```python
from build123d import *

# Parameters (mm, degrees)
ESQUISSE1_R                  = 1.5
BOSS_EXTRU_1_DEPTH           = 3
CONG_1_R                     = 5
ESQUISSE2_W                  = 9
ESQUISSE2_H                  = 9
BOSS_EXTRU_2_DEPTH           = 7
ESQUISSE3_R                  = 2.5
ENL_V_MAT_EXTRU_1_DEPTH      = 7
ESQUISSE6_R                  = 1.5
ENL_V_MAT_EXTRU_2_DEPTH      = 52.639313998
ENL_V_MAT_EXTRU_3_DEPTH      = 3
CONG_2_R                     = 5
CONG_5_R                     = 2
CONG_7_R                     = 4
CONG_8_R                     = 4
CONG_10_R                    = 1
CONG_11_R                    = 3
ESQUISSE8_R                  = 2.5
ENL_V_MAT_EXTRU_4_DEPTH      = 1
ENL_V_MAT_EXTRU_5_DEPTH      = 58.566971538
ENL_V_MAT_EXTRU_5_DEPTH_BACK = 58.566971538
ESQUISSE9_R                  = 14.5


# Some blends are built 0.0001 mm under size
with BuildPart() as part:
    # Esquisse1 → Boss.-Extru.1 (new body)
    with BuildSketch(Plane(origin=(0, 0, 0), x_dir=(1, 0, 0), z_dir=(0, 1, 0))):
        with BuildLine():
            Line((-43.062018769, 37.558204832), (-43.062018769, 28.558204832))
            Line((-43.062018769, 28.558204832), (-9.062018769, 28.558204832))
            Line((-9.062018769, 28.558204832), (-9.062018769, 16.558204832))
            Line((-9.062018769, 16.558204832), (-10.400687943, 16.558204832))
            ThreePointArc((-10.400687943, 16.558204832), (-22.504500987, 1.48048564), (-34.608314032, 16.558204832))
            Line((-34.608314032, 16.558204832), (-43.062018769, 16.558204832))
            Line((-43.062018769, 16.558204832), (-43.062018769, 7.558204832))
            ThreePointArc((-43.062018769, 7.558204832), (-21.562018769, -5.358424695), (-0.062018769, 7.558204832))
            Line((-0.062018769, 7.558204832), (-0.062018769, 37.558204832))
            Line((-0.062018769, 37.558204832), (-43.062018769, 37.558204832))
        make_face()
        with Locations(Location((-38.562018769, 33.058204832, 0), (0, 0, 270))):
            Circle(ESQUISSE1_R, mode=Mode.SUBTRACT)
        with Locations(Location((-4.452018769, 33.058204832, 0), (0, 0, 270))):
            Circle(ESQUISSE1_R, mode=Mode.SUBTRACT)
        with Locations(Location((-38.562018769, 12.058204832, 0), (0, 0, 270))):
            Circle(ESQUISSE1_R, mode=Mode.SUBTRACT)
        with Locations(Location((-4.452018769, 12.058204832, 0), (0, 0, 270))):
            Circle(ESQUISSE1_R, mode=Mode.SUBTRACT)
    extrude(amount=BOSS_EXTRU_1_DEPTH)

    # Congé1
    # the kernel refuses this fillet: 5 mm, written as the material it takes off along each edge
    with BuildSketch(Plane(origin=(-10.400687943, -7.42198732, -16.558204832), x_dir=(1, 0, 0), z_dir=(0, 1, 0))) as cong_1_piece_1:
        with BuildLine():
            CenterArc((5.289036165, -3.065061278), CONG_1_R, 142.192371197, 36.541408835)
            Line((0.290257108, -2.954571735), (0.190281527, -2.952361944))
            ThreePointArc((0.190281527, -2.952361944), (0.1343702, -1.478342768), (-0.09763425, -0.021622979))
            Line((-0.09763425, -0.021622979), (0, 0.1))
            ThreePointArc((0, 0.1), (0.669334587, 0.1), (1.259661834, 0.061301226))
            Line((1.259661834, 0.061301226), (1.338669174, 0))
        make_face()
    extrude(amount=17.84397464, mode=Mode.SUBTRACT)
    with BuildSketch(Plane(origin=(-34.608314032, -12.844953969, -16.558204832), x_dir=(-0.04210418762599367, 0, 0.9991132255076776), z_dir=(0, 1, 0))) as cong_1_piece_2:
        with BuildLine():
            CenterArc((5.211896668, -4.922904418), CONG_1_R, 100.074581009, 82.338524577)
            Line((0.216330541, -5.133425356), (0.116419218, -5.137635775))
            Line((0.116419218, -5.137635775), (-0.099911323, -0.004210419))
            Line((-0.099911323, -0.004210419), (0.017492994, 0.098458088))
            ThreePointArc((0.017492994, 0.098458088), (2.168623487, -0.091152287), (4.31975398, 0.098458088))
            Line((4.31975398, 0.098458088), (4.337246974, 0))
        make_face()
    extrude(amount=28.689907938, mode=Mode.SUBTRACT)
    with BuildSketch(Plane(origin=(-43.062018769, -12.5, -37.558204832), x_dir=(0, 0, 1), z_dir=(0, 1, 0))) as cong_1_piece_3:
        with BuildLine():
            CenterArc((CONG_1_R, CONG_1_R), CONG_1_R, 180, 90)
            Line((0, CONG_1_R), (-CONG_1_R * 0.02, CONG_1_R))
            Line((-CONG_1_R * 0.02, CONG_1_R), (-CONG_1_R * 0.02, -CONG_1_R * 0.02))
            Line((-CONG_1_R * 0.02, -CONG_1_R * 0.02), (CONG_1_R, -CONG_1_R * 0.02))
            Line((CONG_1_R, -CONG_1_R * 0.02), (CONG_1_R, 0))
        make_face()
    extrude(amount=28, mode=Mode.SUBTRACT)
    with BuildSketch(Plane(origin=(-43.062018769, -12.5, -28.558204832), x_dir=(0, 0, -1), z_dir=(0, 1, 0)), Plane(origin=(-43.062018769, -12.5, -16.558204832), x_dir=(1, 0, 0), z_dir=(0, 1, 0))) as cong_1_piece_4:
        with BuildLine():
            CenterArc((CONG_1_R, -CONG_1_R), CONG_1_R, 90, 90)
            Line((0, -CONG_1_R), (-CONG_1_R * 0.02, -CONG_1_R))
            Line((-CONG_1_R * 0.02, -CONG_1_R), (-CONG_1_R * 0.02, CONG_1_R * 0.02))
            Line((-CONG_1_R * 0.02, CONG_1_R * 0.02), (CONG_1_R, CONG_1_R * 0.02))
            Line((CONG_1_R, CONG_1_R * 0.02), (CONG_1_R, 0))
        make_face()
    extrude(amount=28, mode=Mode.SUBTRACT)
    with BuildSketch(Plane(origin=(-43.062018769, -3.711884718, -7.558204832), x_dir=(0, 0, -1), z_dir=(0, 1, 0))) as cong_1_piece_5:
        with BuildLine():
            CenterArc((1.32357905, -5), CONG_1_R, 90, 31.501244596)
            Line((-1.28900638, -0.736855929), (-1.341258088, -0.651593047))
            ThreePointArc((-1.341258088, -0.651593047), (-0.699748478, -0.271785559), (-0.046958464, 0.088288746))
            Line((-0.046958464, 0.088288746), (0, 0.1))
            Line((0, 0.1), (1.32357905, 0.1))
            Line((1.32357905, 0.1), (1.32357905, 0))
        make_face()
    extrude(amount=10.423769437, mode=Mode.SUBTRACT)

    # Esquisse2 → Boss.-Extru.2 (add)
    with BuildSketch(Plane(origin=(0, 3, 0), x_dir=(1, 0, 0), z_dir=(0, 1, 0))):
        with Locations((-4.562018769, 15.758204832)):
            Rectangle(ESQUISSE2_W, ESQUISSE2_H)
    extrude(amount=BOSS_EXTRU_2_DEPTH)

    # Esquisse3 → Enlèv. mat.-Extru.1 (cut)
    with BuildSketch(Plane(origin=(0, 10, 0), x_dir=(1, 0, 0), z_dir=(0, 1, 0))):
        with Locations((-4.452018769, 12.058204832)):
            Circle(ESQUISSE3_R)
    extrude(amount=-ENL_V_MAT_EXTRU_1_DEPTH, mode=Mode.SUBTRACT)

    # Esquisse6 → Enlèv. mat.-Extru.2 (cut, through all)
    with BuildSketch(Plane.ZY.offset(9.062018769)):
        with Locations((-15.758204832, 6.5)):
            Circle(ESQUISSE6_R)
    extrude(amount=-ENL_V_MAT_EXTRU_2_DEPTH, mode=Mode.SUBTRACT)

    # Esquisse7 → Enlèv. mat.-Extru.3 (cut)
    with BuildSketch(Plane.ZY.offset(9.062018769)):
        Polygon((-14.114150837, 3.649195471), (-12.467308691, 6.49839026), (-14.111362685, 9.349194789), (-17.402258826, 9.350804529), (-19.049100972, 6.50160974), (-17.405046978, 3.650805211), align=None)
    extrude(amount=-ENL_V_MAT_EXTRU_3_DEPTH, mode=Mode.SUBTRACT)

    # Congé2
    cong_2_edges = [part.edges().sort_by_distance(p)[0] for p in [
        (-0.062018769, 1.5, -37.558204832),
        (-9.062018769, 1.5, -28.558204832),
    ]]
    fillet(cong_2_edges, radius=CONG_2_R)

    # Congé5
    cong_5_edges = [part.edges().sort_by_distance(p)[0] for p in [
        (-4.562018769, 3, -20.258204832),
    ]]
    fillet(cong_5_edges, radius=CONG_5_R)

    # Congé7
    cong_7_edges = [part.edges().sort_by_distance(p)[0] for p in [
        (-4.562018769, 10, -20.258204832),
    ]]
    fillet(cong_7_edges, radius=CONG_7_R)

    # Congé8
    cong_8_edges = [part.edges().sort_by_distance(p)[0] for p in [
        (-7.941290697, 10, -11.258204832),
    ]]
    fillet(cong_8_edges, radius=CONG_8_R - 0.0001)  # a hair under: the kernel refuses the full size

    # Congé10
    cong_10_edges = [part.edges().sort_by_distance(p)[0] for p in [
        (-7.941290697, 3, -11.258204832),
        (-1.072746841, 3, -11.258204832),
    ]]
    fillet(cong_10_edges, radius=CONG_10_R)

    # Congé11
    cong_11_edges = [part.edges().sort_by_distance(p)[0] for p in [
        (-0.062018769, 1.5, -7.558204832),
    ]]
    fillet(cong_11_edges, radius=CONG_11_R)

    # Esquisse8 → Enlèv. mat.-Extru.4 (cut)
    with BuildSketch(Plane(origin=(0, 3, 0), x_dir=(1, 0, 0), z_dir=(0, 1, 0))):
        with Locations(Location((-4.452018769, 12.058204832, 0), (0, 0, 270))):
            Circle(ESQUISSE8_R)
    extrude(amount=-ENL_V_MAT_EXTRU_4_DEPTH, mode=Mode.SUBTRACT)

    # Esquisse9 → Enlèv. mat.-Extru.5 (cut, two sides: drawn at the far end of the back side and taken through both)
    with BuildSketch(Plane(origin=(0, 3, 0), x_dir=(1, 0, 0), z_dir=(0, 1, 0)).offset(-ENL_V_MAT_EXTRU_5_DEPTH_BACK)):
        with Locations((-21.507018769, 15.558204832)):
            Circle(ESQUISSE9_R)
    extrude(amount=ENL_V_MAT_EXTRU_5_DEPTH + ENL_V_MAT_EXTRU_5_DEPTH_BACK, mode=Mode.SUBTRACT)


solid = part.part
```
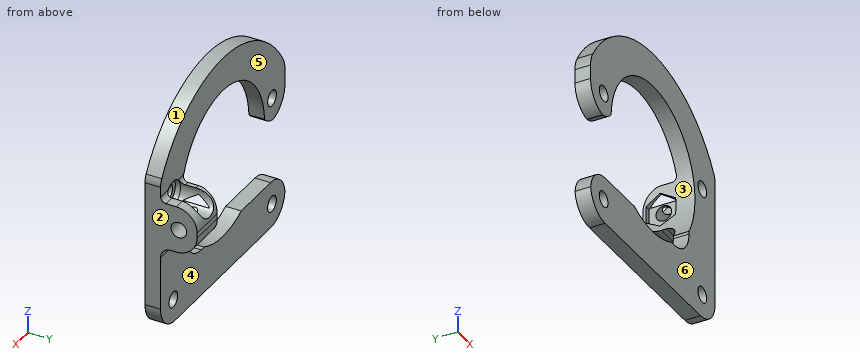
Can you work these out from the model? Positions are in its coordinate system, mm. Face numbers are marked on the shaded views. A direction names the side the tool comes from. Coordinates: 2 decimals unless noted, no trailing zeros. Write each loop counter-clockwise with the first axis right and the second up, starting at its lowest first coordinate (ties: lowest second). Pieces come first, ordered by that corner, then holes. Notation, with made-up numbers: M 86.5,11.5 L 120.5,11.5 A24 cw 120.5,23.5 Z; hole C 81.25,50.5 d11. An arc over 180 degrees is marked long. Write item = value, one per line. Start each with the question number.
Q1. Thinking about a two-plate mould opening in Z: for the marked faces 1, 2 and 3, which applies, released by +Z, released by -Z, zero draft, split by the parting line, or undercut?
Q2. On a 3-axis mill with a long thin cutter (end or side, diameter ignored), from which of +Z, -Z, +X, -X, +Y, -Y can I reach the whole of each face in a straight line? I mean the marked faces 4, 5 and 6. Say none if no direction works.
Q3. If we section it at C-C, the plane y = 1.5: Write out the boundary of the cut face in (x, z).
Q4. If we section it at B-B, the plane x = -30.5: Write out the boundary of the cut face in (y, z).
Q5. I'm going to push flat-ended pins straight in: pin 1 (4 mm diameter, centred on x = -4.45, z = -12.06, fed in from -Y); pin 2 (1 mm diameter, centred on y = 5, z = -24, fed in from -X); pin 3 (0.7 mm diameter, centred on x = -7.5, y = 5, fed in from +Z); pin 4 (5 mm diameter, centred on y = 3, z = -32, fed in from -X). Where does each tip first touch, or does it pass through?
Q6. If we section it at A-A, the plane z = -2: Write out the boundary of the cut face in (x, y).
Q7. If I drill on L1, parallel to Y at x = -10, z = 1.5; L2, parallel to X at y = 3.25, z = -14; L3, parallel to Z at x = -25, y = 1.25, over which ranges is the centre line in solid material (lowest first)? Write a range as [from, to].
Check sheet entries:
q1.face_1 = released by +Z
q1.face_2 = zero draft
q1.face_3 = undercut
q2.face_4 = -Z, +X, -X, +Y
q2.face_5 = +Z, -X, +Y
q2.face_6 = +Z, -Z, +X, -X, -Y
q3.outline = M -43.06,-11.56 A5 ccw -38.9,-16.49 A5 ccw -35.99,-14.86 A14.5 cw long -9.06,-23 L -9.06,-23.56 A5 cw -14.06,-28.56 L -15.08,-28.56 A14.5 cw -27.93,-28.56 L -38.06,-28.56 A5 ccw -43.04,-33.06 A5 ccw -38.06,-37.56 L -5.06,-37.56 A5 ccw -0.06,-32.56 L -0.06,-8.33 A3 ccw -0.46,-6.83 A24.35 ccw -42.33,-6.27 A5 ccw -43.06,-8.88 Z; hole C -38.56,-33.06 d3; hole C -38.56,-12.06 d3; hole C -4.45,-33.06 d3; hole C -4.45,-12.06 d3
q4.outline = M 0,-37.56 L 3,-37.56 L 3,-28.56 L 0,-28.56 Z; M 0,-4.18 L 3,-4.18 L 3,3.66 L 0,3.66 Z
q5.pin_1 = 0
q5.pin_2 = through
q5.pin_3 = -11.26
q5.pin_4 = -43.04
q6.outline = M -39,0 L -26.65,0 L -26.65,3 L -39,3 Z; M -16.37,0 L -4.12,0 L -4.12,3 L -16.37,3 Z
q7.L1 = [0, 3]
q7.L2 = [-7.09, -6.03], [-2.88, -0.06]
q7.L3 = [-37.56, -29.63], [-1.49, 5.11]
